Geometry: see drawing. Coordinates: mm, zero at the bounding-box minimum. Give positions to 0.01 mm unless a question says otherwise; leave off trailing zeros. Loops run counter-clockwise (first coordinate to the right, second up) from the corner with the lowest first, then second, coordinate; pieces in that order, holes last. Notation, with made-up numbers: M 1.5,1 L 9.5,1 A21 ccw 9.5,35 Z; hole C -28,31 d2. An arc over 180 degrees is marked long. Use CSV: the item, a comma, the result in double quotes. Start each with the question number.
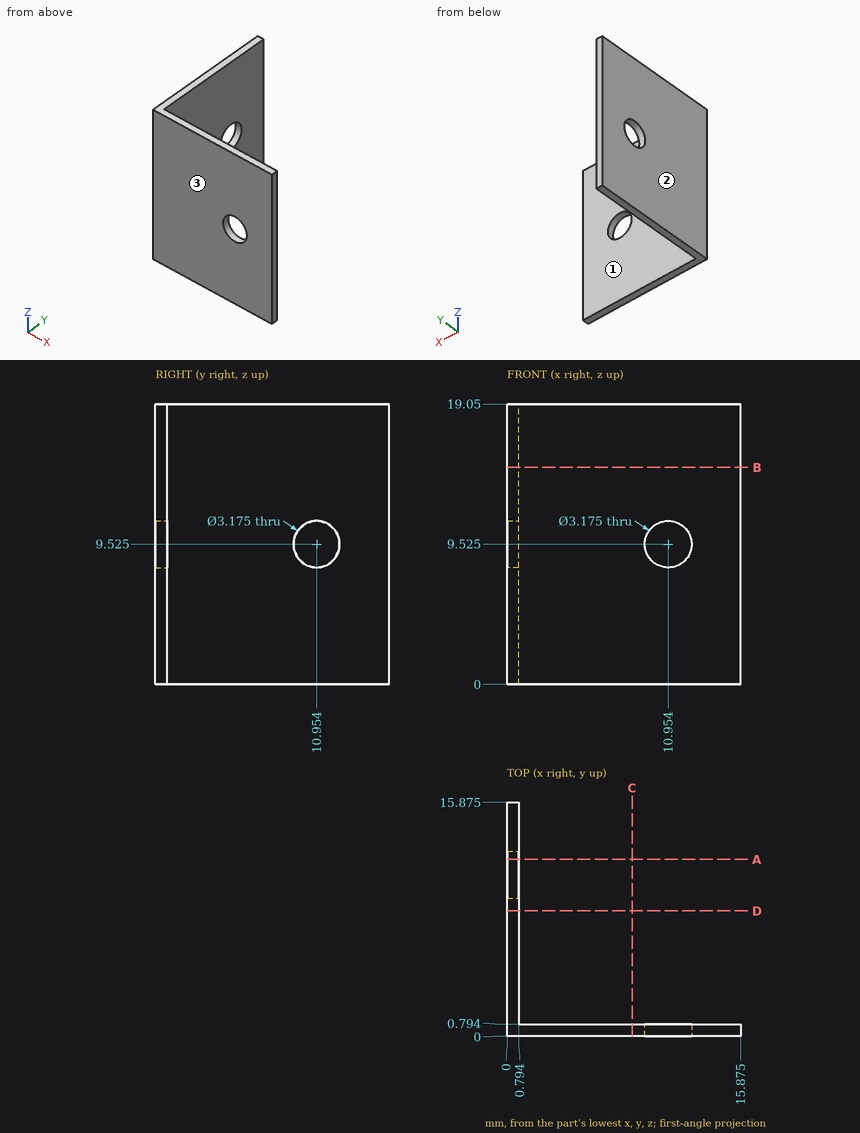
Item 1: Section B-B (z = 14.75). Output: boundary loops of the cut face in (x, y) (1 decimal).
Item 2: Material intervals for line 1 (X direction, y = 1, z = 16), sorted ascending.
Item 3: Mould query, pull axis Y, two halves, no side actions, for the marked faces 1, 2 and 3. Classes: +Y half, -Y half, draft (parallel to the pull), parting line (faces both ways), or undercut.
Item 4: Section C-C (x = 8.5). Output: boundary loops of the cut face in (y, z).
Item 5: First-contact query: pin 1 Ø2 at (y, z) = (8.5, 6.5) entering from +X; pin 2 Ø1 at (y, z) = (9, 15) entering from -X; pin 3 Ø4 at (x, z) = (5.5, 2.5) entering from +Y. Flat tips, straight axial feed; report the tip coordinate or a pass-through.
Item 6: Section A-A (y = 12). Output: boundary loops of the cut face in (x, z), then the cut area to 3 significant figures.
Recorded:
1,outline,"M 0,0 L 15.9,0 L 15.9,0.8 L 0.8,0.8 L 0.8,15.9 L 0,15.9 Z"
2,line 1,"0 to 0.79"
3,face 1,"+Y half"
3,face 2,"draft"
3,face 3,"-Y half"
4,outline,"M 0,0 L 0.79,0 L 0.79,19.05 L 0,19.05 Z"
5,pin 1,"x = 0.79"
5,pin 2,"x = 0"
5,pin 3,"y = 0.79"
6,outline,"M 0,0 L 0.79,0 L 0.79,8.33 L 0,8.33 Z; M 0,10.72 L 0.79,10.72 L 0.79,19.05 L 0,19.05 Z"
6,area,"13.2 mm²"
